Here's how the part is built. I have some questions about the finished solid (model axes, mm). Face numbers are marked on the shaded views. A direction names the side the tool comes from. Round coordinates to 2 decimals unless told otherwise and drop trailing zeros. Write each loop counter-clockwise with the first axis right and the second up, starting at its lowest first coordinate (ties: lowest second). Pieces come first, ordered by that corner, then holes. Notation, with made-up numbers: (38.5, 54) -> (73.5, 54) arc R15 cw to (73.5, 78) -> close; hole circle Ø5 at (29, 3). An arc over 180 degrees is marked (long way). Put each result on its own line as item: value. Start each with the question number.
1. Which directions (+Z, -Z, +X, -X, +Y, -Y) give clear straight access to the entire face, cutting with the end or side of a thin tool? Please do the marked faces 4 and 5.
2. Suppose I cut it at B-B (y = 0). Please give me the cut outline in (x, z) (1 decimal).
3. I need wall thicknesses on probe 1 along X at (y, z) = (0, 8.25) (3 decimals); probe 2 along Z at (x, y) = (0, 5.05); probe 3 along Z at (x, y) = (0, 4.6). Which ranges of each line are inside material? Lowest first, please. Write a range as from..to.
4. We'd pull the mould along Z, two halves only. Please class the marked faces 1, 2 and 3: +Z half, -Z half, draft (parallel to the pull), parting line (faces both ways), or undercut.
5. Suppose I cut it at C-C (z = 3). Please give me the cut outline in (x, y).
6. For pin 1 (5 mm diameter, centred on x = -5, z = 2, fed in from +Y); pin 2 (5 mm diameter, centred on y = 6, z = 10.5, fed in from -X); pin 3 (3 mm diameter, centred on x = 0, z = 10, fed in from +Y); pin 4 (1 mm diameter, centred on y = 5.5, z = 2, fed in from -X), each with a flat end and sliding along its axis, tell me the tip position at first contact or that it passes through.
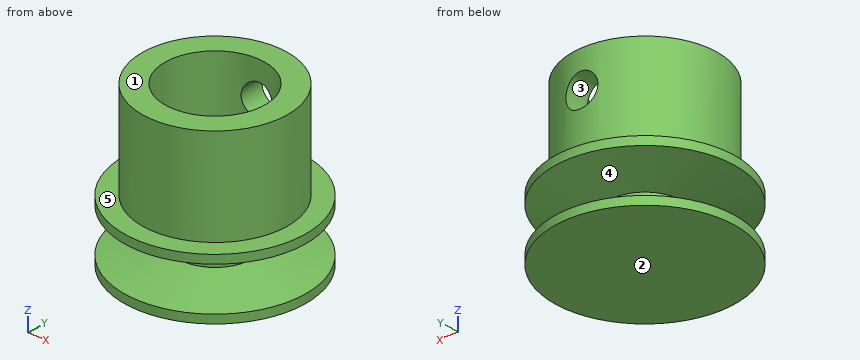
Autodesk Fusion 360 part; units mm, degrees
sketch "Esquisse1" plane through (0, 0, 0) normal (0, 0, 1) x (1, 0, 0)
  circle A0 centre (0, 0) radius 7.5
  dimension "d1" = 15
extrude "Extrusion1" add sketch "Esquisse1" along normal blind 5
sketch "Esquisse2" plane through (0, 0, 0) normal (0, 1, 0) x (1, 0, 0)
sketch "Esquisse3" plane through (0, 0, 0) normal (0, 1, 0) x (1, 0, 0)
  line L0 (3, -3.5) -> (8.18, -4.4134)
  line L1 (8.18, -4.4134) -> (8.18, -0.5866)
  line L2 (8.18, -0.5866) -> (3, -1.5)
  line L3 (3, -1.5) -> (3, -3.5)
  line L4 (0, -1.75) -> (0, -22.5)
  dimension "d4" = 2
  dimension "d6" = 1.5
  dimension "d7" = 100
  dimension "d8" = 100
  dimension "d9" = 3
revolve "Révolution1" cut sketch "Esquisse3" angle 360 about axis through (0, 0, 1.75) along (0, 0, 1)
sketch "Esquisse4" plane through (0, 0, 5) normal (0, 0, 1) x (-1, 0, 0)
  circle A0 centre (0, 0) radius 7.5
  circle A1 centre (0, 0) radius 6
  dimension "d11" = 12
extrude "Extrusion2" add sketch "Esquisse4" along normal blind 8 contours A1
sketch "Esquisse5" plane through (0, 0, 13) normal (0, 0, 1) x (-1, 0, 0)
  circle A0 centre (0, 0) radius 6
  circle A1 centre (0, 0) radius 4.125
  dimension "d14" = 8.25
sketch "Esquisse6" plane through (0, 0, 13) normal (0, 0, 1) x (1, 0, 0)
extrude "Extrusion3" cut sketch "Esquisse5" against normal blind 7 contours A1
sketch "Esquisse7" plane through (0, 0, 0) normal (0, 1, 0) x (1, 0, 0)
  circle A0 centre (0, -10) radius 1.35
  line L0 (-6, -13) -> (6, -13)
  dimension "d17" = 2.7
  dimension "d18" = 3
extrude "Extrusion4" cut sketch "Esquisse7" along normal blind 15.5
Verdict:
1. face 4: none
1. face 5: +Z
2. outline: (-7.5, 0) -> (7.5, 0) -> (7.5, 0.7) -> (3, 1.5) -> (3, 3.5) -> (7.5, 4.3) -> (7.5, 5) -> (6, 5) -> (6, 13) -> (4.1, 13) -> (4.1, 6) -> (-4.1, 6) -> (-4.1, 13) -> (-6, 13) -> (-6, 5) -> (-7.5, 5) -> (-7.5, 4.3) -> (-3, 3.5) -> (-3, 1.5) -> (-7.5, 0.7) -> close
3. probe 1: x = -6..-4.125, 4.125..6
3. probe 2: z = 0..1.14, 3.86..8.65, 11.35..13
3. probe 3: z = 0..1.22, 3.78..8.65, 11.35..13
4. face 1: +Z half
4. face 2: -Z half
4. face 3: undercut
5. outline: circle Ø6 at (0, 0)
6. pin 1: stops at y = 6.93
6. pin 2: stops at x = -4.87
6. pin 3: stops at y = 6
6. pin 4: passes through
